```python
from build123d import *

# Parameters (mm, degrees)
SKETCH1_R               = 22.5
BOSS_EXTRUDE1_DEPTH     = 36
SKETCH1_3_R             = 2.25
CUT_EXTRUDE1_DEPTH      = 10
SKETCH2_R               = 33.5
BOSS_EXTRUDE2_DEPTH     = 3
SKETCH3_R               = 3.1
CUT_EXTRUDE2_DEPTH      = 10
CUT_EXTRUDE2_DEPTH_BACK = 3


with BuildPart() as part:
    # Sketch1 → Boss-Extrude1 (new body)
    with BuildSketch(Plane.XY):
        Circle(SKETCH1_R)
    extrude(amount=BOSS_EXTRUDE1_DEPTH)

    # Sketch1_3 → Cut-Extrude1 (cut)
    with BuildSketch(Plane.XY):
        with Locations((0, 15)):
            Circle(SKETCH1_3_R)
        with Locations((15, 0)):
            Circle(SKETCH1_3_R)
        with Locations((0, -15)):
            Circle(SKETCH1_3_R)
        with Locations((-15, 0)):
            Circle(SKETCH1_3_R)
    extrude(amount=CUT_EXTRUDE1_DEPTH, mode=Mode.SUBTRACT)

    # Sketch2 → Boss-Extrude2 (add)
    with BuildSketch(Plane.XY.offset(36)):
        Circle(SKETCH2_R)
    extrude(amount=BOSS_EXTRUDE2_DEPTH)

    # Sketch3 → Cut-Extrude2 (cut, two sides)
    with BuildSketch(Plane(origin=(0, 0, 36), x_dir=(-1, 0, 0), z_dir=(0, 0, -1))) as cut_extrude2_sk:
        with Locations((0, 12.5)):
            Circle(SKETCH3_R)
        with Locations((12.5, 0)):
            Circle(SKETCH3_R)
        with Locations((0, -12.5)):
            Circle(SKETCH3_R)
        with Locations((-12.5, 0)):
            Circle(SKETCH3_R)
    extrude(amount=CUT_EXTRUDE2_DEPTH, mode=Mode.SUBTRACT)
    extrude(cut_extrude2_sk.sketch, amount=-CUT_EXTRUDE2_DEPTH_BACK, mode=Mode.SUBTRACT)


solid = part.part
```
CAD build for the part. Positions are in the model's coordinates, mm. A direction names the side the tool comes from. Round coordinates to 2 decimals unless told otherwise and drop trailing zeros. Write each loop counter-clockwise with the first axis right and the second up, starting at its lowest first coordinate (ties: lowest second). Pieces come first, ordered by that corner, then holes.
Item 1: Drill centre lines: L1, parallel to Y at x = 0, z = 32; L2, parallel to Y at x = 0, z = 3.25; L3, parallel to Z at x = 25, y = -12. Where is each one in solid material? Low to high.
Filled in:
L1: y = -22.5 to -15.6, -9.4 to 9.4, 15.6 to 22.5
L2: y = -22.5 to -17.25, -12.75 to 12.75, 17.25 to 22.5
L3: z = 36 to 39
Item 2: Band-saw the part on B-B on z = 27. Write the cut outline in (x, y).
Filled in:
outline: circle Ø45 at (0, 0); hole circle Ø6.2 at (-12.5, 0); hole circle Ø6.2 at (0, -12.5); hole circle Ø6.2 at (0, 12.5); hole circle Ø6.2 at (12.5, 0)
Item 3: Band-saw the part on C-C on x = 14. Write the cut outline in (y, z), then the cut area to 3 significant figures.
Filled in:
outline: (-30.43, 36) - (-17.61, 36) - (-17.61, 0) - (-2.02, 0) - (-2.02, 10) - (2.02, 10) - (2.02, 0) - (17.61, 0) - (17.61, 36) - (30.43, 36) - (30.43, 39) - (2.71, 39) - (2.71, 26) - (-2.71, 26) - (-2.71, 39) - (-30.43, 39) - close
area: 1,340 mm2
Item 4: Band-saw the part on D-D on z = 2. Write the cut outline in (x, y), then the cut area to 3 significant figures.
Filled in:
outline: circle Ø45 at (0, 0); hole circle Ø4.5 at (-15, 0); hole circle Ø4.5 at (0, -15); hole circle Ø4.5 at (0, 15); hole circle Ø4.5 at (15, 0)
area: 1,530 mm2
Item 5: Drop flat-ended pins along their axis: pin 1 Ø3.5 at (x, y) = (12.5, 0) entering from +Z; pin 2 Ø1 at (x, y) = (-23.5, -0.5) entering from -Z; pin 3 Ø4 at (x, z) = (10.5, 6.5) entering from +Y. Give the stop position or say it passes through.
Filled in:
pin 1: stops at z = 26
pin 2: stops at z = 36
pin 3: stops at y = 20.83
Item 6: Mould opens along X. For faces 4 (the flat face through (22, -7, 36)), 5 (the cylindrical face through (-0.488, 12.804, 4.93)), 6 (the cylindrical face through (-7.262, -32.703, 37.479)) say: released by +X, released by -X, zero draft, split by the parting line, or undercut.
Filled in:
face 4: zero draft
face 5: undercut
face 6: split by the parting line
Item 7: Band-saw the part on A-A on y = 0. Write the cut outline in (x, z).
Filled in:
outline: (-33.5, 36) - (-22.5, 36) - (-22.5, 0) - (-17.25, 0) - (-17.25, 10) - (-12.75, 10) - (-12.75, 0) - (12.75, 0) - (12.75, 10) - (17.25, 10) - (17.25, 0) - (22.5, 0) - (22.5, 36) - (33.5, 36) - (33.5, 39) - (15.6, 39) - (15.6, 26) - (9.4, 26) - (9.4, 39) - (-9.4, 39) - (-9.4, 26) - (-15.6, 26) - (-15.6, 39) - (-33.5, 39) - close
Item 8: Tool access for faces 1 (the flat face through (0, 0, 39)), 2 (the flat face through (0, 15, 10)), 3 (the flat face through (0, 13, 26)): list every direction of +Z, -Z, +X, -X, +Y, -Y with a clear straight run to the whole face (end or side of a thin tool).
Filled in:
face 1: +Z, +X, -X, +Y, -Y
face 2: -Z
face 3: +Z
